The model under review builds one solid part; all positions refer to its coordinate system, in mm. Face numbers are marked on the shaded views. A direction names the side the tool comes from. Round coordinates to 2 decimals unless told otherwise and drop trailing zeros. Order: outer loops, then holes, each group sorted by start corner. A loop starts at its lowest first (then second) coordinate and runs counter-clockwise, first axis right, second up. Notation, with made-up numbers: M 77.5,7.5 L 113.5,7.5 A9 cw 113.5,24.5 Z; hole C 67,36.5 d8. An arc over 180 degrees is marked long. One line per item, written item: value. Start each with the question number.
from build123d import *

# Parameters (mm, degrees)
F1_DEPTH = 3.175
F3_DEPTH = 6.35


with BuildPart() as f1:
    # F0 (on Front) → F1 (new body)
    with BuildSketch(Plane.XZ):
        Polygon((5.260512, 12.7), (-5.260512, 12.7), (-12.7, 5.260512), (-12.7, -5.260512), (-5.260512, -12.7), (5.260512, -12.7), (12.7, -5.260512), (12.7, 5.260512), align=None)
    extrude(amount=-F1_DEPTH)

    # F2 (on face) → F3 (join)
    with BuildSketch(Plane.XZ):
        Polygon((5.260512, -12.7), (12.7, -5.260512), (12.7, 5.260512), (5.260512, 12.7), (-5.260512, 12.7), (-12.7, 5.260512), (-12.7, -5.260512), (-5.260512, -12.7), align=None)
        Polygon((-3.886145, 0), (-1.943072, 3.3655), (1.943072, 3.3655), (3.886145, 0), (1.943072, -3.3655), (-1.943072, -3.3655), align=None, mode=Mode.SUBTRACT)
    extrude(amount=F3_DEPTH)


solid = f1.part
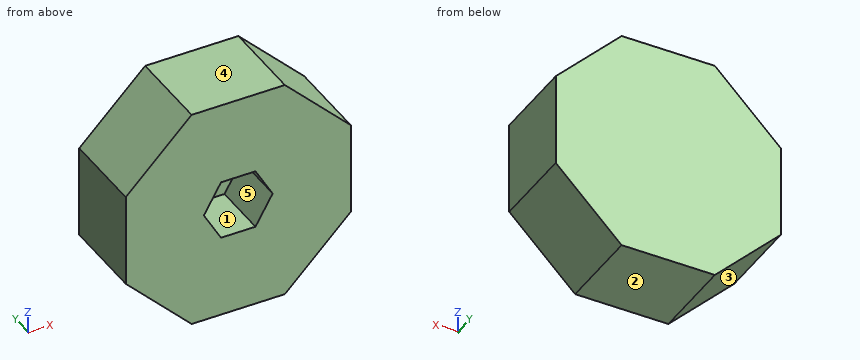
Item 1: Consider section B-B, the plane y = 0.75. Give the boundary of the cut face in (x, z), then the cut area to 3 significant figures.
Item 2: Wall thickness on L1, parallel to Z at x = -1.75, y = -3.5; L2, parallel to X at y = -5, z = -2.5; L3, parallel to Y at x = -1.25, z = 3 (3 decimals): over which ranges is each line inside the solid? List them lowest first.
Item 3: Consider section C-C, the plane x = -2.5. Give the boundary of the cut face in (y, z) (3 decimals).
Item 4: Consider section A-A, the plane y = -3.5. Give the boundary of the cut face in (x, z), then the cut area to 3 significant figures.
Item 5: The part is to be moulded in two halves that separate along Z. For the marked faces 3, 4 and 5, say which applies: pulls with the +Z half, pulls with the -Z half, needs draft (parallel to the pull), parting line crosses it, or undercut.
Item 6: Consider section D-D, the plane z = 10.5. Give the boundary of the cut face in (x, y) (3 decimals).
Item 7: Machinability: for the marked faces 1 and 2, which of the approach directions +Z, -Z, +X, -X, +Y, -Y give a long, thin tool a straight path to every point of the face, cutting with its end or side? Answer none if there is none.
Computed:
1. outline: M -12.7,-5.26 L -5.26,-12.7 L 5.26,-12.7 L 12.7,-5.26 L 12.7,5.26 L 5.26,12.7 L -5.26,12.7 L -12.7,5.26 Z
1. area: 534 mm^2
2. L1: z = -12.7 to -3.37, 3.37 to 12.7
2. L2: x = -12.7 to -2.44, 2.44 to 12.7
2. L3: y = 0 to 3.175
3. outline: M -6.35,-12.7 L 3.175,-12.7 L 3.175,12.7 L -6.35,12.7 L -6.35,2.401 L 0,2.401 L 0,-2.401 L -6.35,-2.401 Z
4. outline: M -12.7,-5.26 L -5.26,-12.7 L 5.26,-12.7 L 12.7,-5.26 L 12.7,5.26 L 5.26,12.7 L -5.26,12.7 L -12.7,5.26 Z; hole M -3.89,0 L -1.94,-3.37 L 1.94,-3.37 L 3.89,0 L 1.94,3.37 L -1.94,3.37 Z
4. area: 495 mm^2
5. face 3: pulls with the -Z half
5. face 4: pulls with the +Z half
5. face 5: undercut
6. outline: M -7.461,-6.35 L 7.461,-6.35 L 7.461,3.175 L -7.461,3.175 Z
7. face 1: -Y
7. face 2: -Z, +X, -X, +Y, -Y
